from build123d import *

# Parameters (mm, degrees)
SKETCH1_W           = 50
SKETCH1_H           = 31.1
BOSS_EXTRUDE1_DEPTH = 11
SKETCH2_W           = 46
SKETCH2_H           = 27.1
CUT_EXTRUDE1_DEPTH  = 9
SKETCH3_R           = 4.25
CUT_EXTRUDE2_DEPTH  = 2
FILLET1_R           = 1
SKETCH4_W           = 50
SKETCH4_H           = 31.1
SKETCH4_W_2         = 48
SKETCH4_H_2         = 29.1
CUT_EXTRUDE3_DEPTH  = 1
SKETCH5_W           = 2.95
SKETCH5_H           = 5
BOSS_EXTRUDE2_DEPTH = 9
SKETCH6_R           = 1.25
CUT_EXTRUDE4_DEPTH  = 8
FILLET2_R           = 2
SKETCH7_W           = 2
SKETCH7_H           = 2
BOSS_EXTRUDE3_DEPTH = 4.3
FILLET3_R           = 1


with BuildPart() as part:
    # Sketch1 → Boss-Extrude1 (new body)
    with BuildSketch(Plane.XY):
        Rectangle(SKETCH1_W, SKETCH1_H)
    extrude(amount=BOSS_EXTRUDE1_DEPTH)

    # Sketch2 → Cut-Extrude1 (cut)
    with BuildSketch(Plane.XY.offset(11)):
        Rectangle(SKETCH2_W, SKETCH2_H)
    extrude(amount=-CUT_EXTRUDE1_DEPTH, mode=Mode.SUBTRACT)

    # Sketch3 → Cut-Extrude2 (cut)
    with BuildSketch(Plane(origin=(0, 0, 0), x_dir=(-1, 0, 0), z_dir=(0, 0, -1))):
        with Locations((8.6, -0.05)):
            Circle(SKETCH3_R)
    extrude(amount=-CUT_EXTRUDE2_DEPTH, mode=Mode.SUBTRACT)

    # Fillet1
    fillet1_edges = [part.edges().sort_by_distance(p)[0] for p in [
        (-4.35, -0.05, 0),
    ]]
    fillet(fillet1_edges, radius=FILLET1_R)

    # Sketch4 → Cut-Extrude3 (cut)
    with BuildSketch(Plane.XY.offset(11)):
        Rectangle(SKETCH4_W, SKETCH4_H)
        Rectangle(SKETCH4_W_2, SKETCH4_H_2, mode=Mode.SUBTRACT)
    extrude(amount=-CUT_EXTRUDE3_DEPTH, mode=Mode.SUBTRACT)

    # Sketch5 → Boss-Extrude2 (add)
    with BuildSketch(Plane.XY.offset(2)):
        with Locations((-21.525, 11.05)):
            Rectangle(SKETCH5_W, SKETCH5_H)
        with Locations((21.525, 11.05)):
            Rectangle(SKETCH5_W, SKETCH5_H)
        with Locations((-21.525, -11.05)):
            Rectangle(SKETCH5_W, SKETCH5_H)
        with Locations((21.525, -11.05)):
            Rectangle(SKETCH5_W, SKETCH5_H)
    extrude(amount=BOSS_EXTRUDE2_DEPTH)

    # Sketch6 → Cut-Extrude4 (cut)
    with BuildSketch(Plane.XY.offset(11)):
        with Locations((-22.025, 11.55)):
            Circle(SKETCH6_R)
        with Locations(Location((22.025, 11.55, 0), (0, 0, 180))):
            Circle(SKETCH6_R)
        with Locations(Location((-22.025, -11.55, 0), (0, 0, 180))):
            Circle(SKETCH6_R)
        with Locations((22.025, -11.55)):
            Circle(SKETCH6_R)
    extrude(amount=-CUT_EXTRUDE4_DEPTH, mode=Mode.SUBTRACT)

    # Fillet2
    fillet2_edges = [part.edges().sort_by_distance(p)[0] for p in [
        (25, -15.55, 5),
        (-25, -15.55, 5),
        (-25, 15.55, 5),
        (25, 15.55, 5),
        (24, -14.55, 10.5),
        (0, -15.55, 0),
        (-24, -14.55, 10.5),
        (-24, 14.55, 10.5),
        (24, 14.55, 10.5),
        (-25, 0, 0),
        (0, 15.55, 0),
        (25, 0, 0),
    ]]
    fillet(fillet2_edges, radius=FILLET2_R)

    # Sketch7 → Boss-Extrude3 (add)
    with BuildSketch(Plane.XY.offset(2)):
        with Locations((-19.05, 12.55)):
            Rectangle(SKETCH7_W, SKETCH7_H)
        with Locations((19.05, 12.55)):
            Rectangle(SKETCH7_W, SKETCH7_H)
        with Locations((19.05, -12.55)):
            Rectangle(SKETCH7_W, SKETCH7_H)
        with Locations((-19.05, -12.55)):
            Rectangle(SKETCH7_W, SKETCH7_H)
    extrude(amount=BOSS_EXTRUDE3_DEPTH)

    # Fillet3
    fillet3_edges = [part.edges().sort_by_distance(p)[0] for p in [
        (23, 8.55, 6.5),
        (20.05, 8.55, 6.5),
        (20.05, 13.55, 8.65),
        (-20.05, 13.55, 8.65),
        (-23, 8.55, 6.5),
        (-23, -8.55, 6.5),
        (-20.05, -8.55, 6.5),
        (-20.05, -13.55, 8.65),
        (20.05, -13.55, 8.65),
        (20.05, -8.55, 6.5),
        (23, -8.55, 6.5),
        (-20.05, 8.55, 6.5),
        (-18.05, -11.55, 4.15),
        (-20.05, -11.55, 4.15),
        (-18.05, 11.55, 4.15),
        (-18.05, 13.55, 4.15),
        (18.05, 13.55, 4.15),
        (18.05, 11.55, 4.15),
        (20.05, 11.55, 4.15),
        (20.05, -11.55, 4.15),
        (18.05, -11.55, 4.15),
        (18.05, -13.55, 4.15),
        (-18.05, -13.55, 4.15),
        (-20.05, 11.55, 4.15),
    ]]
    fillet(fillet3_edges, radius=FILLET3_R - 0.0001)  # a hair under: the kernel refuses the full size


solid = part.part
Can you work these out from the model? Positions are in its coordinate system, mm. A direction names the side the tool comes from. Coordinates: 2 decimals unless noted, no trailing zeros. Write each loop counter-clockwise with the first axis right and the second up, starting at its lowest first coordinate (ties: lowest second). Pieces come first, ordered by that corner, then holes. Notation, with made-up numbers: (-25.5, 73) -> (-12.5, 73) arc R4 ccw to (-12.5, 80) -> close; hole circle Ø3 at (26, -11). An arc over 180 degrees is marked (long way). Write item = value, one per line.
(1) Imagine slicing it at A-A (x = -8.6). Please give me the cut outline in (y, z).
Verdict:
outline = (-15.55, 2) arc R2 ccw to (-13.55, 0) -> (-5.3, 0) arc R1 ccw to (-4.3, 1) -> (-4.3, 2) -> (-13.55, 2) -> (-13.55, 11) -> (-14.55, 11) -> (-14.55, 10) -> (-15.55, 10) -> close; (4.2, 1) arc R1 ccw to (5.2, 0) -> (13.55, 0) arc R2 ccw to (15.55, 2) -> (15.55, 10) -> (14.55, 10) -> (14.55, 11) -> (13.55, 11) -> (13.55, 2) -> (4.2, 2) -> close
(2) Imagine slicing it at B-B (y = -0.05). Please give me the cut outline in (x, z), and give its area (3 significant figures).
Verdict:
outline = (-25, 2) arc R2 ccw to (-23, 0) -> (-13.85, 0) arc R1 ccw to (-12.85, 1) -> (-12.85, 2) -> (-23, 2) -> (-23, 11) -> (-24, 11) -> (-24, 10) -> (-25, 10) -> close; (-4.35, 1) arc R1 ccw to (-3.35, 0) -> (23, 0) arc R2 ccw to (25, 2) -> (25, 10) -> (24, 10) -> (24, 11) -> (23, 11) -> (23, 2) -> (-4.35, 2) -> close
area = 115 mm^2
(3) Thinking about a two-plate mould opening in X: for faces 3 (the face through (-23, 0, 7)), 4 (the face through (19, 12, 6.3)), 5 (the face through (0, 0, 0)), 6 (the face through (25, 0, 6)), which applies, +X half, -X half, draft (parallel to the pull), parting line (faces both ways), or undercut?
Verdict:
face_3 = undercut
face_4 = undercut
face_5 = draft
face_6 = +X half
(4) On a 3-axis mill with a long thin cutter (end or side, diameter ignored), from which of +Z, -Z, +X, -X, +Y, -Y can I reach the whole of each face in a straight line? I mean faces 1 (the face through (22.715, -8.249, 6.563)), 2 (the face through (-4, 14, 11)). Say none if no direction works.
Verdict:
face_1 = +Z
face_2 = +Z, +X, -X, +Y, -Y
(5) For pin 1 (4 mm diameter, centred on x = -7, y = 5, fed in from +Z); pin 2 (1.2 mm diameter, centred on x = 22, y = -11.5, fed in from +Z); pin 3 (0.8 mm diameter, centred on y = -5, z = 10.5, fed in from +X), each with a flat end and sliding along its axis, tell me the tip position at first contact or that it passes through.
Verdict:
pin_1 = 2
pin_2 = 3
pin_3 = 24
(6) If I drill on probe 1 along X at (y, z) = (11.5, 7.25); probe 2 along Y at (x, z) = (15.5, 4.25); probe 3 along X at (y, z) = (-3.5, 7.25), over which ranges is the centre line in solid material (lowest first)?
Verdict:
probe_1 = -25 to -23.27, -20.78 to -20.05, 20.05 to 20.78, 23.27 to 25
probe_2 = -15.55 to -13.55, 13.55 to 15.55
probe_3 = -25 to -23, 23 to 25
(7) Imagine slicing it at D-D (z = 5). State how many separate pieces and enclosed holes the cut face has, and give its area (3 significant figures).
Verdict:
separate_pieces = 1
enclosed_holes = 5
area = 361 mm^2
(8) Imagine slicing it at C-C (x = 3.5). Please give me the cut outline in (y, z).
Verdict:
outline = (-15.55, 2) arc R2 ccw to (-13.55, 0) -> (13.55, 0) arc R2 ccw to (15.55, 2) -> (15.55, 10) -> (14.55, 10) -> (14.55, 11) -> (13.55, 11) -> (13.55, 2) -> (-13.55, 2) -> (-13.55, 11) -> (-14.55, 11) -> (-14.55, 10) -> (-15.55, 10) -> close
